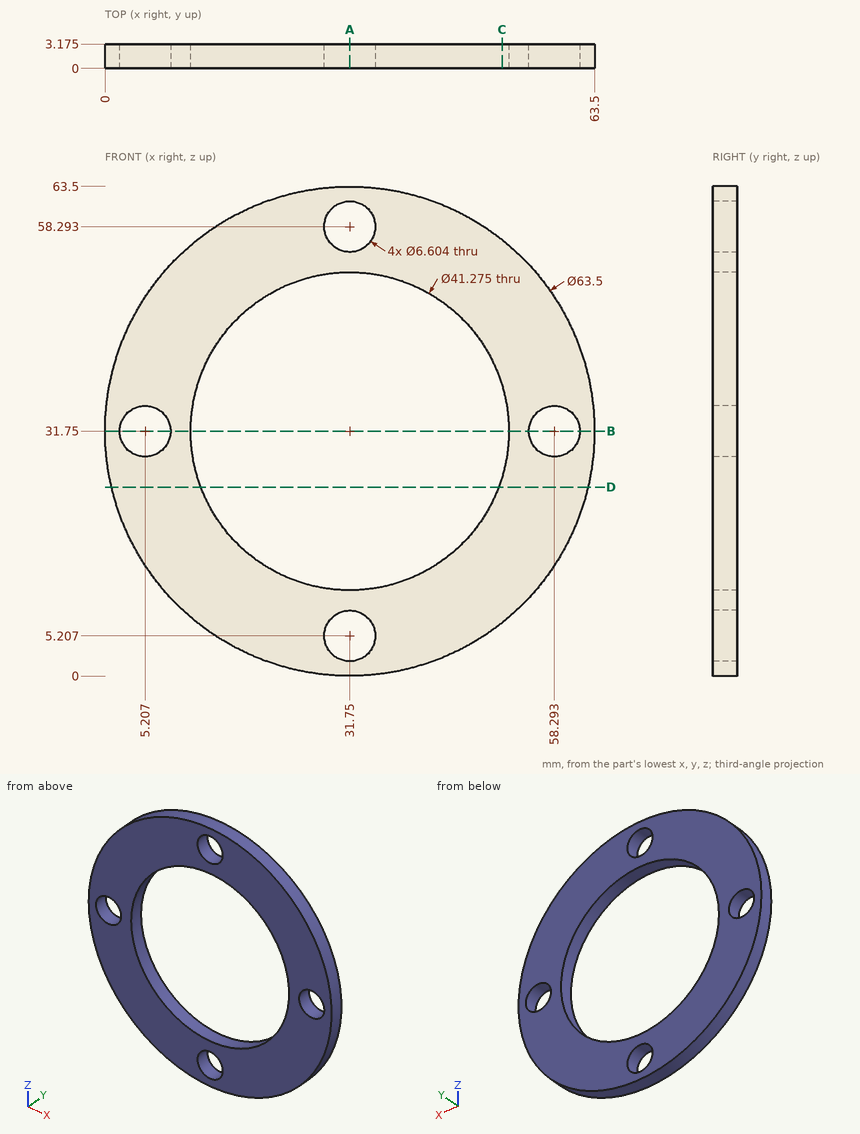
For this review, use the dimensioned drawing (mm, ordinates from the lowest corner) and the shaded views. Round coordinates to 2 decimals unless told otherwise and drop trailing zeros. Order: outer loops, then holes, each group sorted by start corner. A loop starts at its lowest first (then second) coordinate and runs counter-clockwise, first axis right, second up. Notation, with made-up numbers: (65, -27) -> (101, -27) arc R15 ccw to (101, -20) -> close; hole circle Ø4 at (-12.5, -38.75). An arc over 180 degrees is marked (long way). Put each result on its own line as item: value.
Q1. Add section C-C on x = 51.5. Write out the cut boundary in (y, z) (3 decimals).
Check result:
outline: (0, 6.89) -> (3.175, 6.89) -> (3.175, 25.763) -> (0, 25.763) -> close; (0, 37.737) -> (3.175, 37.737) -> (3.175, 56.61) -> (0, 56.61) -> close
Q2. For probe 1 along Z at (x, y) = (31.75, 2.55) (1 decimal); probe 2 along Z at (x, y) = (31, 2); probe 3 along X at (y, z) = (2.8, 49), list the stretches that pass through material, from the lowest coordinate up. Write a range as [from, to].
Check result:
probe 1: [0, 1.9], [8.5, 11.1], [52.4, 55], [61.6, 63.5]
probe 2: [0.01, 1.99], [8.42, 11.13], [52.37, 55.08], [61.51, 63.49]
probe 3: [5.09, 20.42], [43.08, 58.41]
Q3. Add section D-D on z = 24.5. Write out the cut boundary in (x, y) (3 decimals).
Check result:
outline: (0.839, 0) -> (12.428, 0) -> (12.428, 3.175) -> (0.839, 3.175) -> close; (51.072, 0) -> (62.661, 0) -> (62.661, 3.175) -> (51.072, 3.175) -> close
Q4. Add section A-A on x = 31.75. Write out the cut boundary in (y, z) (1 decimal), plus the area to 3 significant figures.
Check result:
outline: (0, 0) -> (3.2, 0) -> (3.2, 1.9) -> (0, 1.9) -> close; (0, 8.5) -> (3.2, 8.5) -> (3.2, 11.1) -> (0, 11.1) -> close; (0, 52.4) -> (3.2, 52.4) -> (3.2, 55) -> (0, 55) -> close; (0, 61.6) -> (3.2, 61.6) -> (3.2, 63.5) -> (0, 63.5) -> close
area: 28.6 mm2
Q5. Add section B-B on z = 31.75. Write out the cut boundary in (x, y) (1 decimal).
Check result:
outline: (0, 0) -> (1.9, 0) -> (1.9, 3.2) -> (0, 3.2) -> close; (8.5, 0) -> (11.1, 0) -> (11.1, 3.2) -> (8.5, 3.2) -> close; (52.4, 0) -> (55, 0) -> (55, 3.2) -> (52.4, 3.2) -> close; (61.6, 0) -> (63.5, 0) -> (63.5, 3.2) -> (61.6, 3.2) -> close
Q6. Insertion check: pin 1 Ø4 at (x, z) = (58.293, 31.75) entering from +Y. The pin has a flat end and moves straight along its axis. Give the tip position at first contact, or say it passes through.
Check result:
pin 1: through
